Autodesk Inventor part; units mm, degrees
ref_plane "Work Plane1" through (29, 0, 0) normal (0, -1, 0) x (1, 0, 0)
ref_plane "YZ Plane" through (0, 0, 0) normal (1, 0, 0) x (0, 1, 0)
ref_plane "XZ Plane" through (0, 0, 0) normal (0, 1, 0) x (-1, 0, 0)
sketch "Sketch1" plane through (0, 0, 0) normal (0, 0, 1) x (1, 0, 0)
  line L0 (0.2879, 0) -> (19.05, 0)
  line L1 (19.05, 0) -> (19.05, 2.413)
  line L2 (19.05, 2.413) -> (2.1084, 2.413)
  line L3 (2.1084, 2.413) -> (0.0001, 2.413)
  line L4 (0.0001, 2.413) -> (0, 2.413)
  line L5 (0, 2.413) -> (0, 4.5847)
  line L6 (0, 4.5847) -> (-2.5654, 4.5847)
  line L7 (-2.5654, 4.5847) -> (-2.5654, 1.8624)
  line L8 (-2.5654, 1.8624) -> (-0.7874, 1.8624)
  line L9 (-0.7874, 1.8624) -> (0.2879, 0)
  line L10 (-6.8885, 0) -> (23.3731, 0)
  line L11 (0, -0.9169) -> (0, 5.5016)
  line L12 (2.1084, 2.413) -> (0, 2.413) construction
  dimension "d1" = 16.9416
  dimension "d2" = 2.1083
  dimension "d3" = 2.5654
  dimension "d4" = 1.778
  dimension "d5" = 60
  dimension "d6" = 4.826
  dimension "d7" = 4.826
  dimension "d8" = 3.7248
  dimension "d9" = 9.1694
  dimension "d26" = 19.05
revolve "Body" add sketch "Sketch1" angle 360 about axis through (0.2879, 0, 0) along (1, 0, 0) contours L9 L11 L3 L2 L1 L0 | L9 L8 L7 L6 L5 L11
sketch "Sketch2" plane through (-2.5654, 0, 0) normal (-1, 0, 0) x (0, 0, 1)
  circle A0 centre (0, 0) radius 1.8624
  line L0 (0, -6.4186) -> (0, 6.4186)
  line L1 (-6.4186, 0) -> (6.4186, 0)
  line L2 (1.8624, 0) -> (0.9312, -1.6129)
  line L3 (0.9312, -1.6129) -> (-0.9312, -1.6129)
  line L4 (-0.9312, -1.6129) -> (-1.8624, 0)
  line L5 (-1.8624, 0) -> (-0.9312, 1.6129)
  line L6 (-0.9312, 1.6129) -> (0.9312, 1.6129)
  line L7 (0.9312, 1.6129) -> (1.8624, 0)
  point P0 (0, 0)
extrude "Slot" add sketch "Sketch2" against normal up to next contours L7 A0 | A0 L2 | L6 L0 A0 | A0 L0 L3 | L0 L6 A0 | A0 L3 L0 | L4 A0 | A0 L5
fillet "Fillet1" radius 2.0574 1 edges at (-2.5654, -4.5847, 0)
thread "Thread"
chamfer "Chamfer1" distance 0.4724 distance2 0.4724 1 edges at (19.05, -2.413, 0) measured on face at (19.05, -1.2173, -0.6389)
ref_plane "Work Plane1" through (29, 0, 0) normal (0, -1, 0) x (1, 0, 0)
fillet "Fillet2" radius 0.1 1 edges at (0.0001, -2.413, 0)
equation "\"d30\" = R"
equation "\"d17\" = RR"
equation "\"d13\" = GEL"
equation "\"d15\" = -0.5 * SPD + 0.5 * GD"
equation "\"d16\" = GUL"
equation "\"d1\" = GEL"
equation "\"d3\" = KOH"
equation "\"d4\" = INTI"
equation "\"d6\" = GD"
equation "\"d7\" = BDM"
equation "\"d8\" = 1.1547 * SW"
equation "\"d9\" = KOD"
equation "\"d26\" = NLG"
equation "\"GD\" = NND"
equation "\"NLG\" = 19.05"
equation "\"GEL\" = 16.9416"
equation "\"KOD\" = 9.1694"
equation "\"KOH\" = 2.5654"
equation "\"INTI\" = 1.778"
equation "\"GAL\" = 2.1082"
equation "\"GUL\" = 0.47244"
equation "\"BDM\" = NND"
equation "\"SW\" = 3.2258"
equation "\"RR\" = 2.0574"
equation "\"SPD\" = 3.88112"
equation "\"R\" = 0.1"
equation "\"TOA\" = 30deg"
equation "\"GD1\" = SPD"
equation "\"THREADDIA\" = 4.826"
equation "\"KOH1\" = 0.508"
equation "\"NND\" = 4.826"
equation "\"E0\" = 3.72593"
properties part number "ANSI B18.3 - No. 10-32 - 3/4, HSBHCSI" material "Steel, Mild"
Source: CAD feature listing. Evaluate the final solid. Frame: model axes, mm. A direction names the side the tool comes from. Give positions to 0.01 mm unless a question says otherwise; leave off trailing zeros. Write each loop counter-clockwise with the first axis right and the second up, starting at its lowest first coordinate (ties: lowest second). Pieces come first, ordered by that corner, then holes.
1. Pull-direction query (Z, two-part tool) for faces 4 (the face through (-0.26, -3.64, 2.79)), 5 (the face through (-1.6, -0.8, 1.4)), 6 (the face through (19.05, 0, 0)); classes: +Z half, -Z half, draft (parallel to the pull), parting line (faces both ways), or undercut.
2. Section query A-A (x = 11.5). Return the cut outline in (y, z), then the cut area to 3 significant figures.
3. Material intervals for line 1 along Z through (x, y) = (2, 0); line 2 along Z through (x, y) = (12.25, 1.25); line 3 along X through (y, z) = (-3.25, -1.75), sorted ascending.
4. First-contact query: pin 1 (4 mm diameter, centred on x = 8, z = -3.5, fed in from +Y); pin 2 (1.5 mm diameter, centred on x = -2, z = -0.5, fed in from -Y); pin 3 (1 mm diameter, centred on y = 0.5, z = -3, fed in from +X). Flat tips, straight axial feed; report the tip coordinate or a pass-through.
5. Access query for faces 1 (the face through (9.21, -1.915, 1.468)), 2 (the face through (-2, 1.613, 0)), 3 (the face through (-2.565, -2, 0)). Directions: +Z, -Z, +X, -X, +Y, -Y. A direction counts if a zero-diameter tool reaches every point of the face in a straight line with its end or side. Return the directions, or none.
Output values:
1. face 4: parting line
1. face 5: undercut
1. face 6: draft
2. outline: circle Ø4.83 at (0, 0)
2. area: 18.3 mm2
3. line 1: z = -2.41 to 2.41
3. line 2: z = -2.06 to 2.06
3. line 3: x = -2.2 to 0
4. pin 1: stops at y = 1.89
4. pin 2: stops at y = -4.43
4. pin 3: stops at x = 0
5. face 1: +X
5. face 2: -X
5. face 3: +Z, -Z, -X, +Y, -Y
